from build123d import *

# Parameters (mm, degrees)
SKETCH_1_W          = 41
SKETCH_1_H          = 31
SKETCH_1_W_2        = 31
SKETCH_1_H_2        = 21
EXTRUDE_1_DEPTH     = 4
SKETCH_2_W          = 41
SKETCH_2_H          = 31
EXTRUDE_1_2_DEPTH   = 1
CUT_EXTRUDE_START   = -5
SKETCH_3_R          = 1.7
CUT_EXTRUDE_1_DEPTH = 2
SKETCH_4_R          = 0.7
CUT_EXTRUDE_2_DEPTH = 26.874698066
FILLET_1_R          = 1
CUT_EXTRUDE_3_DEPTH = 4
EXTRUDE_2_DEPTH     = 2


with BuildPart() as part:
    # 草图1 → Extrude 1 (new body)
    with BuildSketch(Plane.XY):
        Rectangle(SKETCH_1_W, SKETCH_1_H)
        Rectangle(SKETCH_1_W_2, SKETCH_1_H_2, mode=Mode.SUBTRACT)
    extrude(amount=EXTRUDE_1_DEPTH)

    # 草图2 → Extrude 1 2 (add)
    with BuildSketch(Plane.XY.offset(4)):
        Rectangle(SKETCH_2_W, SKETCH_2_H)
    extrude(amount=EXTRUDE_1_2_DEPTH)

    # 草图3 → 切除-拉伸1 (cut)
    with BuildSketch(Plane(origin=(0, 0, 0), x_dir=(-1, 0, 0), z_dir=(0, 0, -1)).offset(CUT_EXTRUDE_START)):
        with Locations(Location((17.5, 12.5, 0), (0, 0, 180))):
            Circle(SKETCH_3_R)
        with Locations(Location((-17.5, 12.5, 0), (0, 0, 180))):
            Circle(SKETCH_3_R)
        with Locations(Location((17.5, -12.5, 0), (0, 0, 180))):
            Circle(SKETCH_3_R)
        with Locations(Location((-17.5, -12.5, 0), (0, 0, 180))):
            Circle(SKETCH_3_R)
    extrude(amount=CUT_EXTRUDE_1_DEPTH, mode=Mode.SUBTRACT)

    # 草图4 → 切除-拉伸2 (cut, through all)
    with BuildSketch(Plane.XY.offset(3)):
        with Locations((17.5, 12.5)):
            Circle(SKETCH_4_R)
        with Locations(Location((-17.5, 12.5, 0), (0, 0, 180))):
            Circle(SKETCH_4_R)
        with Locations(Location((17.5, -12.5, 0), (0, 0, 180))):
            Circle(SKETCH_4_R)
        with Locations((-17.5, -12.5)):
            Circle(SKETCH_4_R)
    extrude(amount=-CUT_EXTRUDE_2_DEPTH, mode=Mode.SUBTRACT)

    # 圆角1
    fillet_1_edges = [part.edges().sort_by_distance(p)[0] for p in [
        (20.5, -15.5, 2.5),
        (-20.5, -15.5, 2.5),
        (-20.5, 15.5, 2.5),
        (20.5, 15.5, 2.5),
    ]]
    fillet(fillet_1_edges, radius=FILLET_1_R)

    # 草图5 → 切除-拉伸3 (cut)
    with BuildSketch(Plane(origin=(0, 0, 0), x_dir=(-1, 0, 0), z_dir=(0, 0, -1))):
        Polygon((-15.5, 10.5), (-15.5, 12.5), (-15.5, 14), (15.5, 14), (15.5, 12.5), (15.5, 10.5), (17.5, 10.5), (19, 10.5), (19, -10.5), (17.5, -10.5), (15.5, -10.5), (15.5, -12.5), (15.5, -14), (-15.5, -14), (-15.5, -12.5), (-15.5, -10.5), (-17.5, -10.5), (-19, -10.5), (-19, 10.5), (-17.5, 10.5), align=None)
    extrude(amount=-CUT_EXTRUDE_3_DEPTH, mode=Mode.SUBTRACT)

    # 草图7 → 凸台-拉伸2 (add)
    with BuildSketch(Plane(origin=(0, 0, 0), x_dir=(-1, 0, 0), z_dir=(0, 0, -1))):
        with BuildLine():
            Line((-20.5, 14.5), (-20.5, -14.5))
            ThreePointArc((-20.5, -14.5), (-20.207106781, -15.207106781), (-19.5, -15.5))
            Line((-19.5, -15.5), (19.5, -15.5))
            ThreePointArc((19.5, -15.5), (20.207106781, -15.207106781), (20.5, -14.5))
            Line((20.5, -14.5), (20.5, 14.5))
            ThreePointArc((20.5, 14.5), (20.207106781, 15.207106781), (19.5, 15.5))
            Line((19.5, 15.5), (-19.5, 15.5))
            ThreePointArc((-19.5, 15.5), (-20.207106781, 15.207106781), (-20.5, 14.5))
        make_face()
        with BuildLine():
            Line((-19.5, 13.5), (-19.5, -13.5))
            ThreePointArc((-19.5, -13.5), (-19.207106781, -14.207106781), (-18.5, -14.5))
            Line((-18.5, -14.5), (18.5, -14.5))
            ThreePointArc((18.5, -14.5), (19.207106781, -14.207106781), (19.5, -13.5))
            Line((19.5, -13.5), (19.5, 13.5))
            ThreePointArc((19.5, 13.5), (19.207106781, 14.207106781), (18.5, 14.5))
            Line((18.5, 14.5), (-18.5, 14.5))
            ThreePointArc((-18.5, 14.5), (-19.207106781, 14.207106781), (-19.5, 13.5))
        make_face(mode=Mode.SUBTRACT)
    extrude(amount=EXTRUDE_2_DEPTH)


solid = part.part
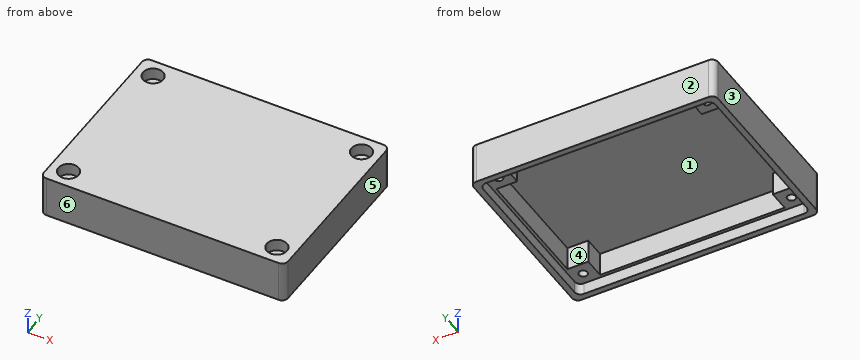
Check sheet for the modelled part. Datum: model origin and axes. Units: mm. Face numbers are marked on the shaded views. A direction names the side the tool comes from. Give positions to 0.01 mm unless a question says otherwise; leave off trailing zeros. Write each loop counter-clockwise with the first axis right and the second up, starting at its lowest first coordinate (ties: lowest second). Pieces come first, ordered by that corner, then holes. Notation, with made-up numbers: (1.5, 77.5) -> (9.5, 77.5) arc R16 ccw to (9.5, 103.5) -> close; hole circle Ø11 at (-39, 83). An arc over 180 degrees is marked (long way). Write item = value, one per line.
Item 1: Sectioned sample at D-D on z = 2. Record the boundary of the cut face in (x, y), and give its area (3 significant figures).
Output:
outline = (-20.5, -14.5) arc R1 ccw to (-19.5, -15.5) -> (19.5, -15.5) arc R1 ccw to (20.5, -14.5) -> (20.5, 14.5) arc R1 ccw to (19.5, 15.5) -> (-19.5, 15.5) arc R1 ccw to (-20.5, 14.5) -> close; hole (-19, -10.5) -> (-15.5, -10.5) -> (-15.5, -14) -> (15.5, -14) -> (15.5, -10.5) -> (19, -10.5) -> (19, 10.5) -> (15.5, 10.5) -> (15.5, 14) -> (-15.5, 14) -> (-15.5, 10.5) -> (-19, 10.5) -> close; hole circle Ø1.4 at (-17.5, -12.5); hole circle Ø1.4 at (-17.5, 12.5); hole circle Ø1.4 at (17.5, -12.5); hole circle Ø1.4 at (17.5, 12.5)
area = 249 mm^2
Item 2: Release check for a two-part mould opening along X. For the marked faces 3, 4, 5 and 6 record: +X half, -X half, draft (parallel to the pull), parting line (faces both ways), or undercut.
Output:
face_3 = -X half
face_4 = undercut
face_5 = +X half
face_6 = draft
Item 3: Scan lines: probe 1 along Y at (x, z) = (17.5, 4.05); probe 2 along Y at (x, z) = (17.5, 1.55); probe 3 along Y at (x, z) = (17.5, 3.85). Record each from-to range of solid material in increasing order. Write a range as from..to.
Output:
probe_1 = -15.5..-14.2, -10.8..10.8, 14.2..15.5
probe_2 = -15.5..-13.2, -11.8..-10.5, 10.5..11.8, 13.2..15.5
probe_3 = -15.5..-14.2, -10.8..-10.5, 10.5..10.8, 14.2..15.5
Item 4: Sectioned sample at B-B on z = -1. Record the boundary of the cut face in (x, y).
Output:
outline = (-20.5, -14.5) arc R1 ccw to (-19.5, -15.5) -> (19.5, -15.5) arc R1 ccw to (20.5, -14.5) -> (20.5, 14.5) arc R1 ccw to (19.5, 15.5) -> (-19.5, 15.5) arc R1 ccw to (-20.5, 14.5) -> close; hole (-19.5, -13.5) arc R1 ccw to (-18.5, -14.5) -> (18.5, -14.5) arc R1 ccw to (19.5, -13.5) -> (19.5, 13.5) arc R1 ccw to (18.5, 14.5) -> (-18.5, 14.5) arc R1 ccw to (-19.5, 13.5) -> close
Item 5: Tool access check on the marked faces 1 and 2. Record the directions out of +Z, -Z, +X, -X, +Y, -Y that give a thin tool (end or side, any length) a straight path to the whole face; none if there is none.
Output:
face_1 = -Z
face_2 = +Z, -Z, +X, -X, +Y
Item 6: Sectioned sample at C-C on x = -17.5. Record the boundary of the cut face in (y, z), and give its area (3 significant figures).
Output:
outline = (-15.5, -2) -> (-14.5, -2) -> (-14.5, 0) -> (-13.2, 0) -> (-13.2, 3) -> (-14.2, 3) -> (-14.2, 5) -> (-15.5, 5) -> close; (-11.8, 0) -> (-10.5, 0) -> (-10.5, 4) -> (10.5, 4) -> (10.5, 0) -> (11.8, 0) -> (11.8, 3) -> (10.8, 3) -> (10.8, 5) -> (-10.8, 5) -> (-10.8, 3) -> (-11.8, 3) -> close; (13.2, 0) -> (14.5, 0) -> (14.5, -2) -> (15.5, -2) -> (15.5, 5) -> (14.2, 5) -> (14.2, 3) -> (13.2, 3) -> close
area = 53.0 mm^2
Item 7: Gauge pin test, flat ends, axial feed: pin 1 (1.1 mm diameter, centred on x = -17.5, y = 12.5, fed in from +Z); pin 2 (2.5 mm diameter, centred on x = 17.5, y = -12.5, fed in from -Z). Record the tip position at first contact, or that the pin passes through.
Output:
pin_1 = through
pin_2 = 0
Item 8: Sectioned sample at A-A on y = 12.5. Record the boundary of the cut face in (x, z), and give its area (3 significant figures).
Output:
outline = (-20.5, -2) -> (-19.5, -2) -> (-19.5, 0) -> (-18.2, 0) -> (-18.2, 3) -> (-19.2, 3) -> (-19.2, 5) -> (-20.5, 5) -> close; (-16.8, 0) -> (-15.5, 0) -> (-15.5, 4) -> (15.5, 4) -> (15.5, 0) -> (16.8, 0) -> (16.8, 3) -> (15.8, 3) -> (15.8, 5) -> (-15.8, 5) -> (-15.8, 3) -> (-16.8, 3) -> close; (18.2, 0) -> (19.5, 0) -> (19.5, -2) -> (20.5, -2) -> (20.5, 5) -> (19.2, 5) -> (19.2, 3) -> (18.2, 3) -> close
area = 63.0 mm^2
